Input: part model. Units: mm. Frame: model coordinates. Round coordinates to 2 decimals unless told otherwise and drop trailing zeros.
(1) Line query: line 1 (Z direction, x = 14.25, y = 5.5); line 2 (Y direction, x = 15.75, z = -1.95); line 3 (Y direction, x = 8, z = -1.1). Output: solid intervals per line, ascending.
(2) First-contact query: pin 1 Ø0.7 at (x, z) = (9, -1) entering from +Y; pin 2 Ø0.7 at (x, y) = (9, -2) entering from -Z; pin 3 Ø0.7 at (x, y) = (19, -1) entering from +Z. Flat tips, straight axial feed; report the tip coordinate or a pass-through.
(3) Cut plane A-A, the plane y = -1.5. Give the number of separate pieces and of enclosed holes in the cut face, and give its area (3 significant figures).
from build123d import *

# Parameters (mm, degrees)
SKETCH1_W              = 20.72
SKETCH1_H              = 2.4
BOSS_EXTRUDE1_DEPTH    = 8.5
SKETCH3_W              = 20.72
SKETCH3_H              = 1.2
CUT_EXTRUDE1_DEPTH     = 0.3
SKETCH4_W              = 0.64
SKETCH4_H              = 0.64
CUT_EXTRUDE2_DEPTH     = 6
CHAMFER2_SIZE          = 0.5
SKETCH5_W              = 0.64
SKETCH5_H              = 0.4
BOSS_EXTRUDE2_DEPTH    = 3.8
CHAMFER3_SIZE          = 1
CHAMFER3_SIZE2         = 0.15838444
CHAMFER3_PART_2_SIZE   = 1
CHAMFER3_PART_2_SIZE2  = 0.15838444
CHAMFER3_PART_3_SIZE   = 1
CHAMFER3_PART_3_SIZE2  = 0.15838444
CHAMFER3_PART_4_SIZE   = 1
CHAMFER3_PART_4_SIZE2  = 0.15838444
CHAMFER3_PART_5_SIZE   = 1
CHAMFER3_PART_5_SIZE2  = 0.15838444
CHAMFER3_PART_6_SIZE   = 1
CHAMFER3_PART_6_SIZE2  = 0.15838444
CHAMFER3_PART_7_SIZE   = 1
CHAMFER3_PART_7_SIZE2  = 0.15838444
CHAMFER3_PART_8_SIZE   = 1
CHAMFER3_PART_8_SIZE2  = 0.15838444
CHAMFER3_PART_9_SIZE   = 1
CHAMFER3_PART_9_SIZE2  = 0.15838444
CHAMFER3_PART_10_SIZE  = 1
CHAMFER3_PART_10_SIZE2 = 0.15838444
CHAMFER3_PART_11_SIZE  = 1
CHAMFER3_PART_11_SIZE2 = 0.15838444
CHAMFER3_PART_12_SIZE  = 1
CHAMFER3_PART_12_SIZE2 = 0.15838444
CHAMFER3_PART_13_SIZE  = 1
CHAMFER3_PART_13_SIZE2 = 0.15838444
CHAMFER3_PART_14_SIZE  = 1
CHAMFER3_PART_14_SIZE2 = 0.15838444
CHAMFER3_PART_15_SIZE  = 1
CHAMFER3_PART_15_SIZE2 = 0.15838444
CHAMFER3_PART_16_SIZE  = 1
CHAMFER3_PART_16_SIZE2 = 0.15838444


with BuildPart() as part:
    # Sketch1 → Boss-Extrude1 (new body)
    with BuildSketch(Plane(origin=(0, 0, 0), x_dir=(1, 0, 0), z_dir=(0, 1, 0))):
        with Locations((10.36, 1.2)):
            Rectangle(SKETCH1_W, SKETCH1_H)
    extrude(amount=BOSS_EXTRUDE1_DEPTH)

    # Sketch3 → Cut-Extrude1 (cut)
    with BuildSketch(Plane.XZ):
        with Locations((10.36, -1.2)):
            Rectangle(SKETCH3_W, SKETCH3_H)
    extrude(amount=-CUT_EXTRUDE1_DEPTH, mode=Mode.SUBTRACT)

    # Sketch4 → Cut-Extrude2 (cut)
    with BuildSketch(Plane(origin=(0, 8.5, 0), x_dir=(1, 0, 0), z_dir=(0, 1, 0))):
        with Locations((4.01, 1.2)):
            Rectangle(SKETCH4_W, SKETCH4_H)
        with Locations((1.47, 1.2)):
            Rectangle(SKETCH4_W, SKETCH4_H)
        with Locations((6.55, 1.2)):
            Rectangle(SKETCH4_W, SKETCH4_H)
        with Locations((9.09, 1.2)):
            Rectangle(SKETCH4_W, SKETCH4_H)
        with Locations((11.63, 1.2)):
            Rectangle(SKETCH4_W, SKETCH4_H)
        with Locations((14.17, 1.2)):
            Rectangle(SKETCH4_W, SKETCH4_H)
        with Locations((16.71, 1.2)):
            Rectangle(SKETCH4_W, SKETCH4_H)
        with Locations((19.25, 1.2)):
            Rectangle(SKETCH4_W, SKETCH4_H)
    extrude(amount=-CUT_EXTRUDE2_DEPTH, mode=Mode.SUBTRACT)

    # Chamfer2
    chamfer2_edges = [part.edges().sort_by_distance(p)[0] for p in [
        (1.79, 8.5, -1.2),
        (1.47, 8.5, -1.52),
        (1.15, 8.5, -1.2),
        (1.47, 8.5, -0.88),
        (4.01, 8.5, -1.52),
        (3.69, 8.5, -1.2),
        (4.01, 8.5, -0.88),
        (4.33, 8.5, -1.2),
        (6.55, 8.5, -1.52),
        (6.23, 8.5, -1.2),
        (6.55, 8.5, -0.88),
        (6.87, 8.5, -1.2),
        (9.09, 8.5, -1.52),
        (8.77, 8.5, -1.2),
        (9.09, 8.5, -0.88),
        (9.41, 8.5, -1.2),
        (11.63, 8.5, -1.52),
        (11.31, 8.5, -1.2),
        (11.63, 8.5, -0.88),
        (11.95, 8.5, -1.2),
        (14.17, 8.5, -1.52),
        (13.85, 8.5, -1.2),
        (14.17, 8.5, -0.88),
        (14.49, 8.5, -1.2),
        (16.71, 8.5, -1.52),
        (16.39, 8.5, -1.2),
        (16.71, 8.5, -0.88),
        (17.03, 8.5, -1.2),
        (19.25, 8.5, -1.52),
        (18.93, 8.5, -1.2),
        (19.25, 8.5, -0.88),
        (19.57, 8.5, -1.2),
    ]]
    chamfer(chamfer2_edges, length=CHAMFER2_SIZE)

    # Sketch5 → Boss-Extrude2 (add)
    with BuildSketch(Plane.XZ.offset(-0.3)):
        with Locations((4.01, -1.2)):
            Rectangle(SKETCH5_W, SKETCH5_H)
        with Locations((1.47, -1.2)):
            Rectangle(SKETCH5_W, SKETCH5_H)
        with Locations((6.55, -1.2)):
            Rectangle(SKETCH5_W, SKETCH5_H)
        with Locations((9.09, -1.2)):
            Rectangle(SKETCH5_W, SKETCH5_H)
        with Locations((11.63, -1.2)):
            Rectangle(SKETCH5_W, SKETCH5_H)
        with Locations((14.17, -1.2)):
            Rectangle(SKETCH5_W, SKETCH5_H)
        with Locations((16.71, -1.2)):
            Rectangle(SKETCH5_W, SKETCH5_H)
        with Locations((19.25, -1.2)):
            Rectangle(SKETCH5_W, SKETCH5_H)
    extrude(amount=BOSS_EXTRUDE2_DEPTH)

    # Chamfer3
    chamfer3_edges = [part.edges().sort_by_distance(p)[0] for p in [
        (1.79, -3.5, -1.2),
    ]]
    chamfer3_side = [part.faces().sort_by_distance(p)[0] for p in [
        (1.79, -1.6, -1.2),
    ]]
    chamfer(chamfer3_edges, length=CHAMFER3_SIZE, length2=CHAMFER3_SIZE2, reference=chamfer3_side[0])

    # Chamfer3 part 2
    chamfer3_part_2_edges = [part.edges().sort_by_distance(p)[0] for p in [
        (1.15, -3.5, -1.2),
    ]]
    chamfer3_part_2_side = [part.faces().sort_by_distance(p)[0] for p in [
        (1.15, -1.6, -1.2),
    ]]
    chamfer(chamfer3_part_2_edges, length=CHAMFER3_PART_2_SIZE, length2=CHAMFER3_PART_2_SIZE2, reference=chamfer3_part_2_side[0])

    # Chamfer3 part 3
    chamfer3_part_3_edges = [part.edges().sort_by_distance(p)[0] for p in [
        (3.69, -3.5, -1.2),
    ]]
    chamfer3_part_3_side = [part.faces().sort_by_distance(p)[0] for p in [
        (3.69, -1.6, -1.2),
    ]]
    chamfer(chamfer3_part_3_edges, length=CHAMFER3_PART_3_SIZE, length2=CHAMFER3_PART_3_SIZE2, reference=chamfer3_part_3_side[0])

    # Chamfer3 part 4
    chamfer3_part_4_edges = [part.edges().sort_by_distance(p)[0] for p in [
        (4.33, -3.5, -1.2),
    ]]
    chamfer3_part_4_side = [part.faces().sort_by_distance(p)[0] for p in [
        (4.33, -1.6, -1.2),
    ]]
    chamfer(chamfer3_part_4_edges, length=CHAMFER3_PART_4_SIZE, length2=CHAMFER3_PART_4_SIZE2, reference=chamfer3_part_4_side[0])

    # Chamfer3 part 5
    chamfer3_part_5_edges = [part.edges().sort_by_distance(p)[0] for p in [
        (6.23, -3.5, -1.2),
    ]]
    chamfer3_part_5_side = [part.faces().sort_by_distance(p)[0] for p in [
        (6.23, -1.6, -1.2),
    ]]
    chamfer(chamfer3_part_5_edges, length=CHAMFER3_PART_5_SIZE, length2=CHAMFER3_PART_5_SIZE2, reference=chamfer3_part_5_side[0])

    # Chamfer3 part 6
    chamfer3_part_6_edges = [part.edges().sort_by_distance(p)[0] for p in [
        (6.87, -3.5, -1.2),
    ]]
    chamfer3_part_6_side = [part.faces().sort_by_distance(p)[0] for p in [
        (6.87, -1.6, -1.2),
    ]]
    chamfer(chamfer3_part_6_edges, length=CHAMFER3_PART_6_SIZE, length2=CHAMFER3_PART_6_SIZE2, reference=chamfer3_part_6_side[0])

    # Chamfer3 part 7
    chamfer3_part_7_edges = [part.edges().sort_by_distance(p)[0] for p in [
        (8.77, -3.5, -1.2),
    ]]
    chamfer3_part_7_side = [part.faces().sort_by_distance(p)[0] for p in [
        (8.77, -1.6, -1.2),
    ]]
    chamfer(chamfer3_part_7_edges, length=CHAMFER3_PART_7_SIZE, length2=CHAMFER3_PART_7_SIZE2, reference=chamfer3_part_7_side[0])

    # Chamfer3 part 8
    chamfer3_part_8_edges = [part.edges().sort_by_distance(p)[0] for p in [
        (9.41, -3.5, -1.2),
    ]]
    chamfer3_part_8_side = [part.faces().sort_by_distance(p)[0] for p in [
        (9.41, -1.6, -1.2),
    ]]
    chamfer(chamfer3_part_8_edges, length=CHAMFER3_PART_8_SIZE, length2=CHAMFER3_PART_8_SIZE2, reference=chamfer3_part_8_side[0])

    # Chamfer3 part 9
    chamfer3_part_9_edges = [part.edges().sort_by_distance(p)[0] for p in [
        (11.31, -3.5, -1.2),
    ]]
    chamfer3_part_9_side = [part.faces().sort_by_distance(p)[0] for p in [
        (11.31, -1.6, -1.2),
    ]]
    chamfer(chamfer3_part_9_edges, length=CHAMFER3_PART_9_SIZE, length2=CHAMFER3_PART_9_SIZE2, reference=chamfer3_part_9_side[0])

    # Chamfer3 part 10
    chamfer3_part_10_edges = [part.edges().sort_by_distance(p)[0] for p in [
        (11.95, -3.5, -1.2),
    ]]
    chamfer3_part_10_side = [part.faces().sort_by_distance(p)[0] for p in [
        (11.95, -1.6, -1.2),
    ]]
    chamfer(chamfer3_part_10_edges, length=CHAMFER3_PART_10_SIZE, length2=CHAMFER3_PART_10_SIZE2, reference=chamfer3_part_10_side[0])

    # Chamfer3 part 11
    chamfer3_part_11_edges = [part.edges().sort_by_distance(p)[0] for p in [
        (13.85, -3.5, -1.2),
    ]]
    chamfer3_part_11_side = [part.faces().sort_by_distance(p)[0] for p in [
        (13.85, -1.6, -1.2),
    ]]
    chamfer(chamfer3_part_11_edges, length=CHAMFER3_PART_11_SIZE, length2=CHAMFER3_PART_11_SIZE2, reference=chamfer3_part_11_side[0])

    # Chamfer3 part 12
    chamfer3_part_12_edges = [part.edges().sort_by_distance(p)[0] for p in [
        (14.49, -3.5, -1.2),
    ]]
    chamfer3_part_12_side = [part.faces().sort_by_distance(p)[0] for p in [
        (14.49, -1.6, -1.2),
    ]]
    chamfer(chamfer3_part_12_edges, length=CHAMFER3_PART_12_SIZE, length2=CHAMFER3_PART_12_SIZE2, reference=chamfer3_part_12_side[0])

    # Chamfer3 part 13
    chamfer3_part_13_edges = [part.edges().sort_by_distance(p)[0] for p in [
        (16.39, -3.5, -1.2),
    ]]
    chamfer3_part_13_side = [part.faces().sort_by_distance(p)[0] for p in [
        (16.39, -1.6, -1.2),
    ]]
    chamfer(chamfer3_part_13_edges, length=CHAMFER3_PART_13_SIZE, length2=CHAMFER3_PART_13_SIZE2, reference=chamfer3_part_13_side[0])

    # Chamfer3 part 14
    chamfer3_part_14_edges = [part.edges().sort_by_distance(p)[0] for p in [
        (17.03, -3.5, -1.2),
    ]]
    chamfer3_part_14_side = [part.faces().sort_by_distance(p)[0] for p in [
        (17.03, -1.6, -1.2),
    ]]
    chamfer(chamfer3_part_14_edges, length=CHAMFER3_PART_14_SIZE, length2=CHAMFER3_PART_14_SIZE2, reference=chamfer3_part_14_side[0])

    # Chamfer3 part 15
    chamfer3_part_15_edges = [part.edges().sort_by_distance(p)[0] for p in [
        (18.93, -3.5, -1.2),
    ]]
    chamfer3_part_15_side = [part.faces().sort_by_distance(p)[0] for p in [
        (18.93, -1.6, -1.2),
    ]]
    chamfer(chamfer3_part_15_edges, length=CHAMFER3_PART_15_SIZE, length2=CHAMFER3_PART_15_SIZE2, reference=chamfer3_part_15_side[0])

    # Chamfer3 part 16
    chamfer3_part_16_edges = [part.edges().sort_by_distance(p)[0] for p in [
        (19.57, -3.5, -1.2),
    ]]
    chamfer3_part_16_side = [part.faces().sort_by_distance(p)[0] for p in [
        (19.57, -1.6, -1.2),
    ]]
    chamfer(chamfer3_part_16_edges, length=CHAMFER3_PART_16_SIZE, length2=CHAMFER3_PART_16_SIZE2, reference=chamfer3_part_16_side[0])


solid = part.part
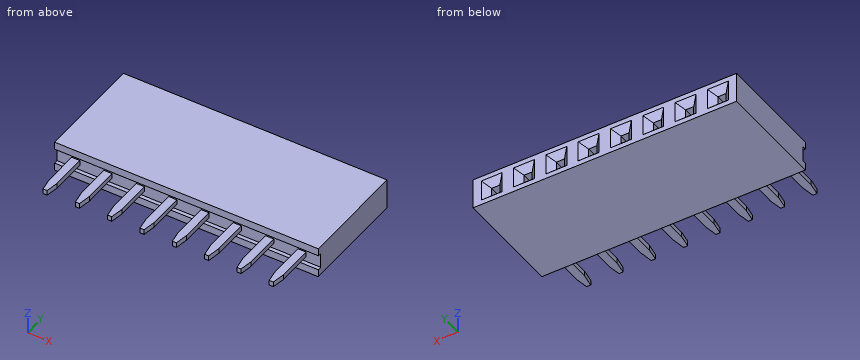
Reported:
1. line 1: z = -2.4 to -1.52, -0.88 to 0
1. line 2: y = 0 to 8.5
1. line 3: y = 0.3 to 8.5
2. pin 1: stops at y = 8.23
2. pin 2: stops at z = -1.4
2. pin 3: stops at z = -1
3. separate pieces: 8
3. enclosed holes: 0
3. area: 2.05 mm2
